Geometry: final body of the model. Coordinates: model frame, mm. A direction names the side the tool comes from. Round coordinates to 2 decimals unless told otherwise and drop trailing zeros. Write each loop counter-clockwise with the first axis right and the second up, starting at its lowest first coordinate (ties: lowest second). Pieces come first, ordered by that corner, then holes. Notation, with made-up numbers: M -13,-31 L 35,-31 A25 cw 35,-7 Z; hole C 48.5,28 d3. An arc over 180 degrees is marked long. Put each result on its own line as item: value. Start each with the question number.
```python
from build123d import *

# Parameters (mm, degrees)
SKETCH_1_W          = 26.5
SKETCH_1_H          = 26.5
SKETCH_1_W_2        = 20.5
SKETCH_1_H_2        = 20.5
EXTRUDE_1_DEPTH     = 50
SKETCH_2_W          = 5.25
SKETCH_2_H          = 32
EXTRUDE_6_DEPTH     = 34
SKETCH_6_R          = 4.5
SKETCH_6_R_2        = 2.15
CUT_EXTRUDE_4_DEPTH = 74.72118081
FILLET_4_R          = 5
FILLET_7_R          = 10
FILLET_8_R          = 10
FILLET_9_R          = 3
SKETCH_7_R          = 2.65
CUT_EXTRUDE_5_DEPTH = 62.899616315
SKETCH_8_R          = 2.65
CUT_EXTRUDE_6_DEPTH = 74.72118081
SKETCH_9_R          = 5
CUT_EXTRUDE_7_DEPTH = 74.72118081


with BuildPart() as part:
    # 草图1 → 凸台-拉伸1 (new body)
    with BuildSketch(Plane.XY):
        Rectangle(SKETCH_1_W, SKETCH_1_H)
        Rectangle(SKETCH_1_W_2, SKETCH_1_H_2, mode=Mode.SUBTRACT)
    extrude(amount=EXTRUDE_1_DEPTH)

    # 草图2 → 凸台-拉伸6 (add)
    with BuildSketch(Plane(origin=(0, 13.25, 0), x_dir=(1, 0, 0), z_dir=(0, 1, 0))):
        with Locations((-10.625, -16)):
            Rectangle(SKETCH_2_W, SKETCH_2_H)
        with Locations((10.625, -16)):
            Rectangle(SKETCH_2_W, SKETCH_2_H)
    extrude(amount=EXTRUDE_6_DEPTH)

    # 草图6 → 切除-拉伸4 (cut, through all)
    with BuildSketch(Plane.ZY.offset(13.25)):
        with Locations((16, 31.25)):
            Circle(SKETCH_6_R)
        with Locations((7.514718626, 39.735281374)):
            Circle(SKETCH_6_R_2)
        with Locations((24.485281374, 39.735281374)):
            Circle(SKETCH_6_R_2)
        with Locations((24.485281374, 22.764718626)):
            Circle(SKETCH_6_R_2)
        with Locations((7.514718626, 22.764718626)):
            Circle(SKETCH_6_R_2)
    extrude(amount=-CUT_EXTRUDE_4_DEPTH, mode=Mode.SUBTRACT)

    # 圆角4
    fillet_4_edges = [part.edges().sort_by_distance(p)[0] for p in [
        (-8, 13.25, 16),
        (-10.625, 13.25, 32),
        (10.625, 13.25, 32),
        (8, 13.25, 16),
    ]]
    fillet(fillet_4_edges, radius=FILLET_4_R)

    # 圆角7
    fillet_7_edges = [part.edges().sort_by_distance(p)[0] for p in [
        (-10.625, 47.25, 0),
        (10.625, 47.25, 0),
    ]]
    fillet(fillet_7_edges, radius=FILLET_7_R)

    # 圆角8
    fillet_8_edges = [part.edges().sort_by_distance(p)[0] for p in [
        (-10.625, 47.25, 32),
        (10.625, 47.25, 32),
    ]]
    fillet(fillet_8_edges, radius=FILLET_8_R)

    # 圆角9
    fillet_9_edges = [part.edges().sort_by_distance(p)[0] for p in [
        (13.25, -13.25, 25),
        (-13.25, -13.25, 25),
    ]]
    fillet(fillet_9_edges, radius=FILLET_9_R)

    # 草图7 → 切除-拉伸5 (cut, through all)
    with BuildSketch(Plane(origin=(0, 13.25, 0), x_dir=(1, 0, 0), z_dir=(0, 1, 0))):
        with Locations(Location((0, -40, 0), (0, 0, 270))):
            Circle(SKETCH_7_R)
    extrude(amount=-CUT_EXTRUDE_5_DEPTH, mode=Mode.SUBTRACT)

    # 草图8 → 切除-拉伸6 (cut, through all)
    with BuildSketch(Plane.ZY.offset(13.25)):
        with Locations((35, 0)):
            Circle(SKETCH_8_R)
        with Locations((15, 0)):
            Circle(SKETCH_8_R)
    extrude(amount=-CUT_EXTRUDE_6_DEPTH, mode=Mode.SUBTRACT)

    # 草图9 → 切除-拉伸7 (cut, through all)
    with BuildSketch(Plane(origin=(13.25, 0, 0), x_dir=(0, 0, -1), z_dir=(1, 0, 0))):
        with Locations(Location((-16, 31.25, 0), (0, 0, 90))):
            Circle(SKETCH_9_R)
    extrude(amount=-CUT_EXTRUDE_7_DEPTH, mode=Mode.SUBTRACT)


solid = part.part
```
1) Access query for faces 5 (the face through (0, 13.25, 30)), 6 (the face through (0, 10.25, 25)), 7 (the face through (-8, 36, 20)). Directions: +Z, -Z, +X, -X, +Y, -Y. A direction counts if a zero-diameter tool reaches every point of the face in a straight line with its end or side. Return the directions, or none.
2) Section A-A, the plane z = 20. Output: boundary loops of the cut face in (x, y).
3) Section C-C, the plane x = 0. Output: boundary loops of the cut face in (y, z).
4) Draft query along Z for faces 1 (the face through (-10.59, 44.4, 28.99)), 2 (the face through (10.66, 44.24, 2.85)), 3 (the face through (-10.25, 0, 25)), 4 (the face through (11.729, 0.117, 32.353)). Return one class per face: +Z half, -Z half, draft (parallel to the pull), parting line (faces both ways), or undercut.
5) Ray query, probe 1 along Z at (x, y) = (-10.25, 23); probe 2 along X at (y, z) = (25, 31.5); probe 3 along Y at (x, z) = (-5.75, 38.5). Return the intervals inside material, ascending.
6) Section D-D, the plane z = 44. Output: boundary loops of the cut face in (x, y), and give its area (3 significant figures).
7) First-contact query: pin 1 (6 mm diameter, centred on x = 0, z = 40, fed in from +Y); pin 2 (12 mm diameter, centred on x = 1, z = 8, fed in from +Y). Flat tips, straight axial feed; report the tip coordinate or a pass-through.
8) Section B-B, the plane y = 0. Output: boundary loops of the cut face in (x, z), and give its area (3 significant figures).
Solved:
1. face 5: +Z, +Y
1. face 6: +Z, -Z
1. face 7: +Z, -Z, +Y
2. outline: M -13.25,-10.25 A3 ccw -10.25,-13.25 L 10.25,-13.25 A3 ccw 13.25,-10.25 L 13.25,28.25 L 8,28.25 L 8,18.25 A5 cw 3,13.25 L -3,13.25 A5 cw -8,18.25 L -8,28.25 L -13.25,28.25 Z; M -13.25,34.25 L -8,34.25 L -8,47.25 L -13.25,47.25 Z; M 8,34.25 L 13.25,34.25 L 13.25,47.25 L 8,47.25 Z; hole M -10.25,-10.25 L 10.25,-10.25 L 10.25,10.25 L -10.25,10.25 Z
3. outline: M -13.25,0 L -10.25,0 L -10.25,37.35 L -13.25,37.35 Z; M -13.25,42.65 L -10.25,42.65 L -10.25,50 L -13.25,50 Z; M 10.25,0 L 13.25,0 L 13.25,37.35 L 10.25,37.35 Z; M 10.25,42.65 L 13.25,42.65 L 13.25,50 L 10.25,50 Z
4. face 1: +Z half
4. face 2: -Z half
4. face 3: draft
4. face 4: undercut
5. probe 1: z = 0 to 5.38, 9.65 to 22.35, 26.62 to 32
5. probe 2: x = -13.25 to -8, 8 to 13.25
5. probe 3: y = -13.25 to -10.25, 10.25 to 13.25
6. outline: M -13.25,-10.25 A3 ccw -10.25,-13.25 L 10.25,-13.25 A3 ccw 13.25,-10.25 L 13.25,13.25 L -13.25,13.25 Z; hole M -10.25,-10.25 L 10.25,-10.25 L 10.25,10.25 L -10.25,10.25 Z
6. area: 278 mm2
7. pin 1: stops at y = 13.25
7. pin 2: stops at y = 15.25
8. outline: M -13.25,0 L -10.25,0 L -10.25,12.35 L -13.25,12.35 Z; M -13.25,17.65 L -10.25,17.65 L -10.25,32.35 L -13.25,32.35 Z; M -13.25,37.65 L -10.25,37.65 L -10.25,50 L -13.25,50 Z; M 10.25,0 L 13.25,0 L 13.25,12.35 L 10.25,12.35 Z; M 10.25,17.65 L 13.25,17.65 L 13.25,32.35 L 10.25,32.35 Z; M 10.25,37.65 L 13.25,37.65 L 13.25,50 L 10.25,50 Z
8. area: 236 mm2
